Work out the finished part from the listing and answer in its coordinate system (mm). Give positions to 0.01 mm unless a question says otherwise; leave off trailing zeros. Write each loop counter-clockwise with the first axis right and the second up, starting at its lowest first coordinate (ties: lowest second). Pieces come first, ordered by that corner, then holes.
1) Determine the mould class of faces 1 (the face through (34.98, 11.02, 11.91)), 2 (the face through (37.852, 11.92, 11.586)), 3 (the face through (35, -12, 0)) for opening direction X: pulls with the +X half, pulls with the -X half, needs draft (parallel to the pull), parting line crosses it, or undercut.
2) Find section A-A (y = 0). Determine the outline of the cut face in (x, z) (3 decimals), plus the area to 3 significant figures.
3) Straight lines are drawn through the part: probe 1 along Y at (x, z) = (0, 15.25) (3 decimals); probe 2 along Z at (x, y) = (12, 36); probe 3 along Y at (x, z) = (3, 7.75). For each, find the intervals that lie inside material, in ascending order.
4) Given pin 1 Ø5 at (x, z) = (3, 22.5) entering from -Y; pin 2 Ø5 at (y, z) = (-15.5, 19) entering from -X; pin 3 Ø8 at (y, z) = (5, 8.5) entering from +X, each flat-ended and moving along its own axis, determine where each tip first touches the part or whether it passes through.
5) Find section C-C (z = 16). Determine the outline of the cut face in (x, y) (3 decimals).
```python
from build123d import *

# Parameters (mm, degrees)
F0_R     = 39.685
F1_DEPTH = 25
F2_R     = 36.675481
F3_DEPTH = 25
F4_R     = 1.5


with BuildPart() as f1:
    # F0 (on Top) → F1 (new body)
    with BuildSketch(Plane.XY):
        Circle(F0_R)
    extrude(amount=F1_DEPTH)

    # F2 (on face) → F3 (cut)
    with BuildSketch(Plane.XY.offset(25)):
        Circle(F2_R)
    extrude(amount=-F3_DEPTH, mode=Mode.SUBTRACT)

    # F4
    f4_edges = [f1.edges().sort_by_distance(p)[0] for p in [
        (-36.675481, 0, 25),
        (-39.685, 0, 25),
    ]]
    fillet(f4_edges, radius=F4_R)


solid = f1.part
```
Results:
1. face 1: undercut
1. face 2: parting line crosses it
1. face 3: needs draft
2. outline: (-39.685, 0) - (-36.675, 0) - (-36.675, 23.5) arc R1.5 ccw to (-38.175, 25) - (-38.185, 25) arc R1.5 ccw to (-39.685, 23.5) - close; (36.675, 0) - (39.685, 0) - (39.685, 23.5) arc R1.5 ccw to (38.185, 25) - (38.175, 25) arc R1.5 ccw to (36.675, 23.5) - close
2. area: 149 mm2
3. probe 1: y = -39.685 to -36.675, 36.675 to 39.685
3. probe 2: z = 0 to 24.98
3. probe 3: y = -39.57 to -36.55, 36.55 to 39.57
4. pin 1: stops at y = -39.68
4. pin 2: stops at x = -37.5
4. pin 3: stops at x = 39.67
5. outline: circle Ø79.37 at (0, 0); hole circle Ø73.351 at (0, 0)
